Read the model definition and answer for the solid it produces. Units are mm, in the model's axes. Face numbers are marked on the shaded views. A direction names the side the tool comes from. Coordinates: 2 decimals unless noted, no trailing zeros. Order: outer loops, then holes, each group sorted by start corner. A loop starts at its lowest first (then second) coordinate and runs counter-clockwise, first axis right, second up. Notation, with made-up numbers: (35, -6.75) -> (50, -6.75) arc R25 cw to (50, 6.25) -> close; hole circle Ø2 at (68, -9.75). An arc over 180 degrees is marked (long way). Use CSV: the item, a comma, the result in double quotes.
```python
from build123d import *

# Parameters (mm, degrees)
F0_W     = 20.5
F0_H     = 6.5
F1_DEPTH = 30
F2_DEPTH = 11
F3_DEPTH = 5.5


with BuildPart() as f1:
    # F0 (on Right) → F1 (new body)
    with BuildSketch(Plane.YZ):
        Polygon((0, 11), (0, 0), (30, 0), (30, 17.5), (9.5, 17.5), (9.5, 11), align=None)
        with Locations((19.75, 20.75)):
            Rectangle(F0_W, F0_H)
        Polygon((9.5, 24), (30, 24), (30, 30), (19, 30), align=None)
        Polygon((0, 18), (0, 11), (9.5, 11), (9.5, 17.5), (9.5, 24), align=None)
    extrude(amount=-F1_DEPTH)

    # F0 (on Right) → F2 (cut)
    with BuildSketch(Plane.YZ):
        Polygon((9.5, 24), (30, 24), (30, 30), (19, 30), align=None)
        Polygon((0, 18), (0, 11), (9.5, 11), (9.5, 17.5), (9.5, 24), align=None)
    extrude(amount=-F2_DEPTH, mode=Mode.SUBTRACT)

    # F0 (on Right) → F3 (cut)
    with BuildSketch(Plane.YZ):
        with Locations((19.75, 20.75)):
            Rectangle(F0_W, F0_H)
    extrude(amount=-F3_DEPTH, mode=Mode.SUBTRACT)


solid = f1.part
```
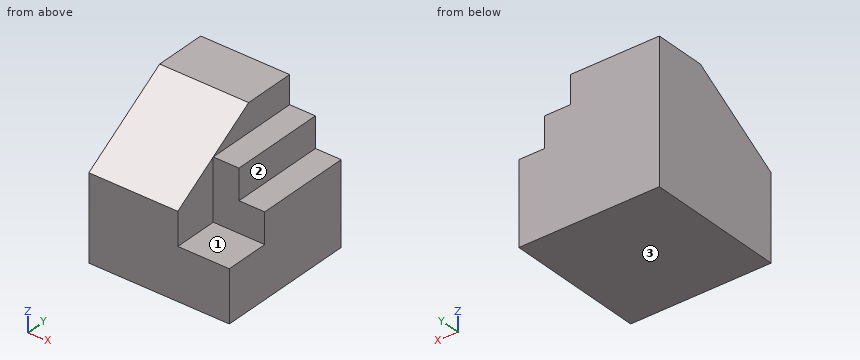
Item 1: Each of these flat-tipped pins is pushed along its axis until it touches: P1, Ø1.8, axis at y = 17.5, z = 25.5, coming from the +X side; P2, Ø3, axis at x = -3.5, y = 23, coming from the +Z side; P3, Ø7.5, axis at y = 6, z = 20.5, coming from the +X side. Where does it stop, or does it pass through?
Return value:
P1,"stops at x = -11"
P2,"stops at z = 17.5"
P3,"stops at x = -5.5"
Item 2: Find section B-B, the plane y = 27.25. Give the vertices of the cut face in (x, z), then the cut area to 3 significant figures.
Return value:
outline,"(-30, 0) -> (0, 0) -> (0, 17.5) -> (-5.5, 17.5) -> (-5.5, 24) -> (-11, 24) -> (-11, 30) -> (-30, 30) -> close"
area,"798 mm^2"
Item 3: Find section D-D, the plane z = 15.25. Give the vertices of the cut face in (x, y), then the cut area to 4 significant figures.
Return value:
outline,"(-30, 0) -> (-11, 0) -> (-11, 9.5) -> (0, 9.5) -> (0, 30) -> (-30, 30) -> close"
area,"795.5 mm^2"
Item 4: Find section A-A, the plane x = -20.5. Give the vertices of the cut face in (y, z), then the cut area to 3 significant figures.
Return value:
outline,"(0, 0) -> (30, 0) -> (30, 30) -> (19, 30) -> (0, 18) -> close"
area,"786 mm^2"
Item 5: Straight lines are drawn through the part: line 1 along Y through (x, z) = (-7.5, 23.5); line 2 along Z through (x, y) = (-7.5, 25.5); line 3 along X through (y, z) = (23.25, 23.25). For each, find the intervals that lie inside material, in ascending order.
Return value:
line 1,"y = 9.5 to 30"
line 2,"z = 0 to 24"
line 3,"x = -30 to -5.5"
Item 6: A tool of negligible diameter and unlimited length cuts with its end or side. For the marked faces 1, 2 and 3, from which of +Z, -Z, +X, -X, +Y, -Y can it reach the whole face along a straight path? Write none if from no direction.
Return value:
face 1,"+Z, +X, -Y"
face 2,"+Z, +X, +Y, -Y"
face 3,"-Z, +X, -X, +Y, -Y"
Item 7: Find section C-C, the plane z = 23. Give the vertices of the cut face in (x, y).
Return value:
outline,"(-30, 7.92) -> (-11, 7.92) -> (-11, 9.5) -> (-5.5, 9.5) -> (-5.5, 30) -> (-30, 30) -> close"
